from build123d import *

# Parameters (mm, degrees)
CUT_EXTRUDE1_DEPTH = 8.92734
CHAMFER1_SIZE      = 0.127
FILLET1_R          = 0.508


with BuildPart() as part:
    # Sketch1 → Revolve1 (revolve)
    with BuildSketch(Plane.XZ):
        Polygon((15.5575, 7.92734), (0, 7.92734), (0, 0), (14.2875, 0), (14.2875, 5.89534), (13.97, 5.89534), (13.97, 6.40334), (15.5575, 6.40334), align=None)
    revolve(axis=Axis((0, 0, 7.92734), (0, 0, -1)))

    # Sketch2 → Cut-Extrude1 (cut, through all)
    with BuildSketch(Plane.XY.offset(7.92734)):
        Polygon((7.332348419, 0), (3.666174209, 6.35), (-3.666174209, 6.35), (-7.332348419, 0), (-3.666174209, -6.35), (3.666174209, -6.35), align=None)
    extrude(amount=-CUT_EXTRUDE1_DEPTH, mode=Mode.SUBTRACT)

    # Chamfer1
    chamfer1_edges = [part.edges().sort_by_distance(p)[0] for p in [
        (-15.5575, 0, 6.40334),
        (-15.5575, 0, 7.92734),
    ]]
    chamfer(chamfer1_edges, length=CHAMFER1_SIZE)

    # Fillet1
    fillet1_edges = [part.edges().sort_by_distance(p)[0] for p in [
        (-14.2875, 0, 0),
    ]]
    fillet(fillet1_edges, radius=FILLET1_R)


solid = part.part
The model under review builds one solid part; all positions refer to its coordinate system, in mm. A direction names the side the tool comes from. Give positions to 0.01 mm unless a question says otherwise; leave off trailing zeros. Write each loop counter-clockwise with the first axis right and the second up, starting at its lowest first coordinate (ties: lowest second). Pieces come first, ordered by that corner, then holes.
1. For P1, Ø1.5, axis at x = 11, z = 2.5, coming from the -Y side; P2, Ø3, axis at x = 12, z = 4, coming from the -Y side; P3, Ø2, axis at y = 0, z = 5, coming from the +X side, all flat-tipped, find the tip position at first contact; note any pin that passes through.
2. Draft analysis for pull direction Y (two halves, no side actions). For faces 1 (the cylindrical face through (-14.274, -0.628, 3.239)), 2 (the flat face through (0, -6.35, 4)), 3 (the flat face through (0, 7, 7.927)), state which applies: +Y half, -Y half, draft (parallel to the pull), parting line (faces both ways), or undercut.
3. Add section B-B, the plane x = 0. Write out the cut boundary in (y, z), plus the area to 3 significant figures.
4. Tool access review of faces 4 (the flat face through (-5.474, 3.219, 4.019)), 5 (the flat face through (2, -14, 6.403)), 6 (the flat face through (-6, 3, 0)): name each direction out of +Z, -Z, +X, -X, +Y, -Y from which nothing blocks a thin tool from reaching the whole face with its end or side.
5. Wall thickness on L1, parallel to Y at x = 1, z = 7.75; L2, parallel to X at y = 4, z = 0.5; L3, parallel to X at y = 3, z = 5.5: over which ranges is each line inside the solid? List them lowest first.
Worked answers:
1. P1: stops at y = -9.95
1. P2: stops at y = -9.69
1. P3: stops at x = 14.29
2. face 1: parting line
2. face 2: undercut
2. face 3: draft
3. outline: (-15.56, 6.53) - (-15.43, 6.4) - (-13.97, 6.4) - (-13.97, 5.9) - (-14.29, 5.9) - (-14.29, 0.51) arc R0.51 ccw to (-13.78, 0) - (-6.35, 0) - (-6.35, 7.93) - (-15.43, 7.93) - (-15.56, 7.8) - close; (6.35, 0) - (13.78, 0) arc R0.51 ccw to (14.29, 0.51) - (14.29, 5.9) - (13.97, 5.9) - (13.97, 6.4) - (15.43, 6.4) - (15.56, 6.53) - (15.56, 7.8) - (15.43, 7.93) - (6.35, 7.93) - close
3. area: 129 mm2
4. face 4: +Z, -Z
4. face 5: none
4. face 6: -Z, +X, -X, +Y, -Y
5. L1: y = -15.53 to -6.35, 6.35 to 15.53
5. L2: x = -13.72 to -5.02, 5.02 to 13.72
5. L3: x = -13.97 to -5.6, 5.6 to 13.97
